Autodesk Inventor part; units mm, degrees
ref_plane "YZ Plane" through (0, 0, 0) normal (1, 0, 0) x (0, 1, 0)
ref_plane "XZ Plane" through (0, 0, 0) normal (0, 1, 0) x (-1, 0, 0)
ref_plane "XY Plane" through (0, 0, 0) normal (0, 0, 1) x (1, 0, 0)
sketch "스케치1" plane through (0, 0, 0) normal (0, 0, 1) x (1, 0, 0)
  line L0 (0, 17.4) -> (0, -17.4) construction
  line L1 (-20, 17.4) -> (-20, -17.4)
  line L2 (20, -17.4) -> (20, 17.4)
  arc A0 (20, 17.4) -> (-20, 17.4) centre (0, 17.4) ccw
  arc A1 (-20, -17.4) -> (20, -17.4) centre (0, -17.4) ccw
  point P0 (0, 0)
  point P1 (0, 0)
  dimension "d0" = 34.8
  dimension "d1" = 40
extrude "돌출1" add sketch "스케치1" along normal blind 25
sketch "스케치2" plane through (0, 0, 25) normal (0, 0, 1) x (1, 0, 0)
  circle A0 centre (0, 19.9) radius 17.5
  arc A1 (20, 17.4) -> (-20, 17.4) centre (0, 17.4) ccw
  point P0 (-6.2408, 3.5506)
  dimension "d4" = 35
  dimension "d26" = 0
extrude "돌출2" add sketch "스케치2" along normal blind 195
sketch "스케치3" plane through (0, 19.9, 220) normal (0, 0, 1) x (1, 0, 0)
  circle A0 centre (0, 0) radius 12.5
  point P0 (0, -19.9)
  dimension "d7" = 25
extrude "돌출3" add sketch "스케치3" along normal blind 34
sketch "스케치5" plane through (0, 0, 0) normal (0, 0, -1) x (-1, 0, 0)
  line L0 (-8.65, 8.75) -> (8.65, 8.75)
  line L1 (8.65, 8.75) -> (8.65, 26.05)
  line L2 (8.65, 26.05) -> (-8.65, 26.05)
  line L3 (-8.65, 26.05) -> (-8.65, 8.75)
  arc A0 (20, 17.4) -> (-20, 17.4) centre (0, 17.4) ccw
  point P0 (0, 0)
  dimension "d10" = 17.3
  dimension "d11" = 17.3
  dimension "d12" = 8.65
  dimension "d13" = 8.65
extrude "돌출4" add sketch "스케치5" along normal blind 19
sketch "스케치6" plane through (-20, -17.4, 0) normal (-1, 0, 0) x (0, 0, 1)
  circle A0 centre (-10, 34.8) radius 3
  line L0 (-19, 26.15) -> (-19, 43.45)
  line L1 (0, 43.45) -> (-19, 43.45)
  circle A1 centre (245, 34.8) radius 3
  line L2 (0, 0) -> (25, 0)
  point P0 (0, 17.4)
  dimension "d16" = 6
  dimension "d17" = 9
  dimension "d18" = 8.65
  dimension "d19" = 255
  dimension "d20" = 34.8
  dimension "d21" = 6
extrude "돌출5" cut sketch "스케치6" against normal through all
sketch "스케치7" plane through (0, 0, 25) normal (0, 0, 1) x (1, 0, 0)
  circle A0 centre (0, -17.4) radius 19
  arc A1 (-20, -17.4) -> (20, -17.4) centre (0, -17.4) ccw
  point P0 (0, 0)
  dimension "d24" = 0
  dimension "d25" = 38
extrude "돌출6" add sketch "스케치7" along normal blind 80
equation "\"d13\" = 0.5 * d10"
properties part number "높이조절 액추에이터_중간" material "알루미늄 6061"
For this review, take the finished solid that the model builds, in its own axes (mm). A direction names the side the tool comes from. Round coordinates to 2 decimals unless told otherwise and drop trailing zeros. Order: outer loops, then holes, each group sorted by start corner. A loop starts at its lowest first (then second) coordinate and runs counter-clockwise, first axis right, second up. Notation, with made-up numbers: (78, -25) -> (94, -25) arc R36 cw to (94, 9) -> close; hole circle Ø8 at (25, 52.5). An arc over 180 degrees is marked (long way). Put each result on its own line as item: value.
Q1. Insertion check: pin 1 Ø8.5 at (x, z) = (3.5, -7.5) entering from -Y; pin 2 Ø6 at (y, z) = (10.5, 62) entering from -X; pin 3 Ø5 at (x, z) = (-10.5, 173) entering from -Y; pin 4 Ø12 at (x, z) = (5.5, 211) entering from +Y. Each pin has a flat end and moves straight along its axis. Give the tip position at first contact, or say it passes through.
Check result:
pin 1: y = 8.75
pin 2: x = -16.29
pin 3: y = 4.34
pin 4: y = 37.4
Q2. Add section A-A on x = 5. Write out the cut boundary in (y, z).
Check result:
outline: (-36.76, 0) -> (8.75, 0) -> (8.75, -19) -> (26.05, -19) -> (26.05, 0) -> (36.76, 0) -> (36.76, 25) -> (36.67, 25) -> (36.67, 220) -> (31.36, 220) -> (31.36, 254) -> (8.44, 254) -> (8.44, 220) -> (3.13, 220) -> (3.13, 25) -> (0.93, 25) -> (0.93, 105) -> (-35.73, 105) -> (-35.73, 25) -> (-36.76, 25) -> close; hole circle Ø6 at (17.4, -10); hole circle Ø6 at (17.4, 245)
Q3. Mouldability with a two-part tool opening along Z and no side actions: class faces 6 (the flat face through (-4, 32, 220)), 7 (the cylindrical face through (-0.175, 20.374, 244.609)), 8 (the flat face through (0, 18, -19)), 9 (the flat face through (-20, 0, 12)) as pulls with the +Z half, pulls with the -Z half, needs draft (parallel to the pull), parting line crosses it, or undercut.
Check result:
face 6: pulls with the +Z half
face 7: undercut
face 8: pulls with the -Z half
face 9: needs draft
Q4. Add section C-C on y = -7. Write out the cut boundary in (x, z), plus the area to 3 significant figures.
Check result:
outline: (-20, 0) -> (20, 0) -> (20, 25) -> (15.9, 25) -> (15.9, 105) -> (-15.9, 105) -> (-15.9, 25) -> (-20, 25) -> close
area: 3,540 mm2
Q5. For probe 1 along Z at (x, y) = (-5, 17); probe 2 along Y at (x, z) = (-0.25, -10); probe 3 along X at (y, z) = (19.5, 126), list the stretches that pass through material, from the lowest coordinate up. Write a range as [from, to].
Check result:
probe 1: [-19, -12.97], [-7.03, 242.03], [247.97, 254]
probe 2: [8.75, 14.4], [20.4, 26.05]
probe 3: [-17.5, 17.5]
Q6. Add section B-B on z = 72.5. Write out the cut boundary in (x, y).
Check result:
outline: circle Ø38 at (0, -17.4); circle Ø35 at (0, 19.9)
Q7. Add section D-D on z = 232.5. Write out the cut boundary in (x, y), plus the area to 3 significant figures.
Check result:
outline: circle Ø25 at (0, 19.9)
area: 491 mm2
Q8. Machinability: for faces 1 (the flat face through (8.65, 16, -7)), 2 (the flat face through (-8.65, 19, -7)), 3 (the cylindrical face through (-3.794, 36.984, 121.135)), 4 (the flat face through (0, 26.05, -9)), 5 (the flat face through (0, -17, 105)), which of the approach directions +Z, -Z, +X, -X, +Y, -Y give a long, thin tool a straight path to every point of the face, cutting with its end or side? Answer none if there is none.
Check result:
face 1: -Z, +X, +Y, -Y
face 2: -Z, -X, +Y, -Y
face 3: +Z
face 4: -Z, +X, -X, +Y
face 5: +Z, +X, -X, -Y
